Geometry check sheet. Reference: the model listing, model coordinates, mm. Face numbers are marked on the shaded views. Round coordinates to 2 decimals unless told otherwise and drop trailing zeros. Loops run counter-clockwise (first coordinate to the right, second up) from the corner with the lowest first, then second, coordinate; pieces in that order, holes last. Notation, with made-up numbers: (3.5, 28) -> (37.5, 28) arc R29 ccw to (37.5, 63) -> close; hole circle Ø11 at (63, -17.75). An arc over 180 degrees is marked (long way). Use one line per item in the form item = value.
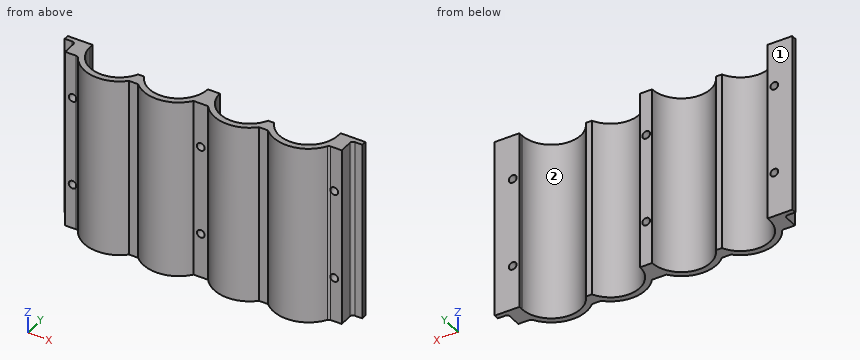
from build123d import *

# Parameters (mm, degrees)
BOSS_EXTRUDE1_DEPTH                  = 60
FILLET1_R                            = 1
F_2_6_START                          = -7
F_2_6_2_6_DIAMETER_HOLE1_OUTLINE_R   = 1.3
F_2_6_2_6_DIAMETER_HOLE1_DEPTH       = 7
F_2_6_START_2                        = -8.425
F_2_6_2_6_DIAMETER_HOLE1_2_OUTLINE_R = 1.3
F_2_6_2_6_DIAMETER_HOLE1_2_DEPTH     = 1.425


# Read off the part's stored shape, not the designer's step: Ø2.6 (2.6) Diameter Hole1
with BuildPart() as part:
    # Sketch1 → Boss-Extrude1 (new body)
    with BuildSketch(Plane.XY):
        with BuildLine():
            Line((0, 0), (8.225, 0))
            Line((8.225, 0), (8.225, -1.25))
            ThreePointArc((8.225, -1.25), (15.833583974, -10.821735736), (26.875, -5.568564576))
            Line((26.875, -5.568564576), (28.875, -5.568564576))
            ThreePointArc((28.875, -5.568564576), (39.831080274, -10.841095968), (47.523441352, -1.425))
            Line((47.523441352, -1.425), (51.476558648, -1.425))
            ThreePointArc((51.476558648, -1.425), (59.168919726, -10.841095968), (70.125, -5.568564576))
            Line((70.125, -5.568564576), (72.125, -5.568564576))
            ThreePointArc((72.125, -5.568564576), (83.166416026, -10.821735736), (90.775, -1.25))
            Line((90.775, -1.25), (90.775, 0))
            Line((90.775, 0), (99, 0))
            Line((99, 0), (99, -1.6))
            Line((99, -1.6), (95.52, -1.6))
            Line((95.52, -1.6), (95.52, -7))
            Line((95.52, -7), (91.282866253, -7))
            ThreePointArc((91.282866253, -7), (82.611549593, -12.957684568), (72.625, -9.647916408))
            Line((72.625, -9.647916408), (69.625, -9.647916408))
            ThreePointArc((69.625, -9.647916408), (60.486058022, -13.046953991), (51.90053193, -8.425))
            Line((51.90053193, -8.425), (47.09946807, -8.425))
            ThreePointArc((47.09946807, -8.425), (38.513941978, -13.046953991), (29.375, -9.647916408))
            Line((29.375, -9.647916408), (26.375, -9.647916408))
            ThreePointArc((26.375, -9.647916408), (16.388450407, -12.957684568), (7.717133747, -7))
            Line((7.717133747, -7), (3.48, -7))
            Line((3.48, -7), (3.48, -1.6))
            Line((3.48, -1.6), (0, -1.6))
            Line((0, -1.6), (0, 0))
        make_face()
    extrude(amount=BOSS_EXTRUDE1_DEPTH)

    # Fillet1
    fillet1_edges = [part.edges().sort_by_distance(p)[0] for p in [
        (95.52, -1.6, 30),
        (91.282866253, -7, 30),
        (7.717133747, -7, 30),
        (3.48, -1.6, 30),
    ]]
    fillet(fillet1_edges, radius=FILLET1_R)

    # Ø2.6 (2.6) Diameter Hole1 outline → Ø2.6 (2.6) Diameter Hole1 (cut)
    with BuildSketch(Plane(origin=(0, 0, 0), x_dir=(1, 0, 0), z_dir=(0, 1, 0)).offset(F_2_6_START)):
        with Locations((93.02, -15)):
            Circle(F_2_6_2_6_DIAMETER_HOLE1_OUTLINE_R)
        with Locations((93.02, -45)):
            Circle(F_2_6_2_6_DIAMETER_HOLE1_OUTLINE_R)
        with Locations((49.5, -15)):
            Circle(F_2_6_2_6_DIAMETER_HOLE1_OUTLINE_R)
        with Locations((49.5, -45)):
            Circle(F_2_6_2_6_DIAMETER_HOLE1_OUTLINE_R)
    f_2_6_2_6_diameter_hole1 = extrude(amount=F_2_6_2_6_DIAMETER_HOLE1_DEPTH, mode=Mode.SUBTRACT)

    # 2.6 _2.6_ Diameter Hole1 2 outline → 2.6 _2.6_ Diameter Hole1 2 (cut)
    with BuildSketch(Plane(origin=(0, 0, 0), x_dir=(1, 0, 0), z_dir=(0, 1, 0)).offset(F_2_6_START_2)):
        with Locations((49.5, -15)):
            Circle(F_2_6_2_6_DIAMETER_HOLE1_2_OUTLINE_R)
        with Locations((49.5, -45)):
            Circle(F_2_6_2_6_DIAMETER_HOLE1_2_OUTLINE_R)
    f_2_6_2_6_diameter_hole1_2 = extrude(amount=F_2_6_2_6_DIAMETER_HOLE1_2_DEPTH, mode=Mode.SUBTRACT)

    # Mirror1: Ø2.6 (2.6) Diameter Hole1, 2.6 _2.6_ Diameter Hole1 2 across plane
    add(f_2_6_2_6_diameter_hole1.mirror(Plane.ZY.offset(-49.5)), mode=Mode.SUBTRACT)
    add(f_2_6_2_6_diameter_hole1_2.mirror(Plane.ZY.offset(-49.5)), mode=Mode.SUBTRACT)


solid = part.part
1. Gauge pin test, flat ends, axial feed: pin 1 (1.6 mm diameter, centred on x = 71, z = 29, fed in from +Y); pin 2 (1.5 mm diameter, centred on x = 28.5, z = 40.5, fed in from -Y); pin 3 (1 mm diameter, centred on y = -0.5, z = 32, fed in from -X); pin 4 (1.2 mm diameter, centred on x = 48.5, z = 30, fed in from +Y) (3 decimals). Record the tip position at first contact, or that the pin passes through.
Return value:
pin_1 = -5.57
pin_2 = -9.65
pin_3 = 0
pin_4 = -1.425
2. Section check C-C (x = 23.5). Record the boundary of the cut face in (y, z), then the cut area to 3 significant figures.
Return value:
outline = (-11.74, 0) -> (-9.42, 0) -> (-9.42, 60) -> (-11.74, 60) -> close
area = 139 mm2
3. Material ranges on line 1 along Z through (x, y) = (49.5, -3.75); line 2 along X through (y, z) = (-3.25, 42); line 3 along X through (y, z) = (-6, 54.5), recorded low to high.
Return value:
line_1 = 0 to 13.7, 16.3 to 43.7, 46.3 to 60
line_2 = 3.48 to 8.43, 47.32 to 51.68, 90.57 to 95.52
line_3 = 3.48 to 9.45, 26.65 to 29.1, 46.3 to 52.7, 69.9 to 72.35, 89.55 to 95.52
4. Mould release check, pull along X, two halves, no side actions. Record for the marked faces 1 and 2: released by +X, released by -X, zero draft, split by the parting line, or undercut.
Return value:
face_1 = zero draft
face_2 = undercut
5. Section check D-D (x = 53.5). Record the boundary of the cut face in (y, z).
Return value:
outline = (-10.14, 0) -> (-7.22, 0) -> (-7.22, 60) -> (-10.14, 60) -> close
6. Section check A-A (x = 93.02). Record the boundary of the cut face in (y, z).
Return value:
outline = (-7, 0) -> (0, 0) -> (0, 13.7) -> (-7, 13.7) -> close; (-7, 16.3) -> (0, 16.3) -> (0, 43.7) -> (-7, 43.7) -> close; (-7, 46.3) -> (0, 46.3) -> (0, 60) -> (-7, 60) -> close
